Input: part model. Units: mm. Frame: model coordinates. Face numbers are marked on the shaded views. A direction names the side the tool comes from. Coordinates: 2 decimals unless noted, no trailing zeros. Order: outer loops, then holes, each group sorted by start corner. A loop starts at its lowest first (then second) coordinate and runs counter-clockwise, first axis right, second up. Notation, with made-up numbers: (40.5, -35.75) -> (47.5, -35.75) arc R15 cw to (47.5, -22.75) -> close; hole circle Ø1 at (51, 28). An arc over 180 degrees is marked (long way). Answer as CSV lines item,"result".
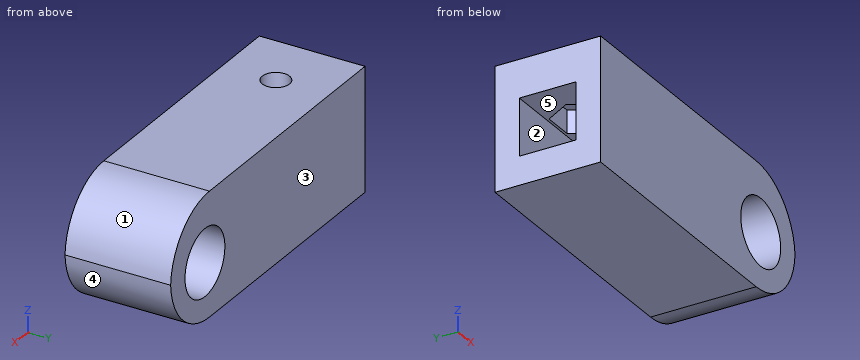
from build123d import *

# Parameters (mm, degrees)
ESBO_O2_R                = 4.1
RESSALTO_EXTRUS_O1_DEPTH = 13
ESBO_O3_W                = 7
ESBO_O3_H                = 7
CORTE_EXTRUS_O1_DEPTH    = 26
CORTE_EXTRUS_O2_DEPTH    = 2.8
ESBO_O10_R               = 1.683661958
CORTE_EXTRUS_O3_DEPTH    = 2.8
FILETE1_R                = 8


with BuildPart() as part:
    # Esboço2 → Ressalto-extrusão1 (new body)
    with BuildSketch(Plane(origin=(0, 0, 0), x_dir=(1, 0, 0), z_dir=(0, 1, 0))):
        Polygon((20, -5), (20, 7), (-20, 7), (-20, -5), (-20, -8.161034979), (20, -8.161034979), align=None)
        with Locations(Location((12.930574096, 0, 0), (0, 0, 90))):
            Circle(ESBO_O2_R, mode=Mode.SUBTRACT)
    extrude(amount=RESSALTO_EXTRUS_O1_DEPTH)

    # Esboço3 → Corte-extrusão1 (cut)
    with BuildSketch(Plane.ZY.offset(20)):
        with Locations((0, 6.5)):
            Rectangle(ESBO_O3_W, ESBO_O3_H)
    extrude(amount=-CORTE_EXTRUS_O1_DEPTH, mode=Mode.SUBTRACT)

    # Esboço7 → Corte-extrusão2 (cut)
    with BuildSketch(Plane(origin=(0, 0, 3.5), x_dir=(-1, 0, 0), z_dir=(0, 0, -1))):
        Polygon((8.882456985, 6.475905175), (10.729977846, 3.275905175), (14.425019569, 3.275905175), (16.272540431, 6.475905175), (14.425019569, 9.675905175), (10.729977846, 9.675905175), align=None)
    extrude(amount=-CORTE_EXTRUS_O2_DEPTH, mode=Mode.SUBTRACT)

    # Esboço10 → Corte-extrusão3 (cut)
    with BuildSketch(Plane(origin=(0, 0, 6.3), x_dir=(-1, 0, 0), z_dir=(0, 0, -1))):
        with Locations((12.577498708, 6.475905175)):
            Circle(ESBO_O10_R)
    extrude(amount=-CORTE_EXTRUS_O3_DEPTH, mode=Mode.SUBTRACT)

    # Filete1
    # the kernel refuses this fillet: 8 mm, written as the material it takes off along each edge
    with BuildSketch(Plane(origin=(20, -20, -7), x_dir=(0, 0, 1), z_dir=(0, 1, 0))) as filete1_piece_1:
        with BuildLine():
            CenterArc((FILETE1_R, -FILETE1_R), FILETE1_R, 90, 90)
            Line((0, -FILETE1_R), (0, 0))
            Line((0, 0), (FILETE1_R, 0))
        make_face()
    extrude(amount=53, mode=Mode.SUBTRACT)
    with BuildSketch(Plane(origin=(20, -20, 8.161034979), x_dir=(0, 0, -1), z_dir=(0, 1, 0))) as filete1_piece_2:
        with BuildLine():
            CenterArc((FILETE1_R, FILETE1_R), FILETE1_R, 180, 90)
            Line((0, FILETE1_R), (0, 0))
            Line((0, 0), (FILETE1_R, 0))
        make_face()
    extrude(amount=53, mode=Mode.SUBTRACT)


solid = part.part
1. Ray query, line 1 along Y through (x, z) = (-3.5, 1); line 2 along Z through (x, y) = (-4, 9.5); line 3 along X through (y, z) = (8.5, 3.75). Return the intervals inside material, ascending.
Findings:
line 1,"y = 0 to 3, 10 to 13"
line 2,"z = -7 to -3.5, 3.5 to 8.16"
line 3,"x = -20 to -15.1, -10.05 to 11.27, 14.59 to 19.15"
2. Cut plane A-A (z = -3). Return the cut outline in (x, y), plus the area to 3 significant figures.
Findings:
outline,"(-20, 0) -> (10.14, 0) -> (10.14, 13) -> (-20, 13) -> (-20, 10) -> (6, 10) -> (6, 3) -> (-20, 3) -> close; (15.73, 0) -> (18.93, 0) -> (18.93, 13) -> (15.73, 13) -> close"
area,"251 mm2"
3. Reachability of the marked faces 4 and 5 from +Z, -Z, +X, -X, +Y, -Y: full face, straight path, thin tool, end or side. Return the list, or none.
Findings:
face 4,"-Z, +X, +Y, -Y"
face 5,"-X"
4. Mould query, pull axis Y, two halves, no side actions, for the marked faces 1, 2 and 3. Classes: released by +Y, released by -Y, zero draft, split by the parting line, or undercut.
Findings:
face 1,"zero draft"
face 2,"undercut"
face 3,"released by +Y"
5. Cut plane B-B (x = -4). Return the cut outline in (y, z), plus the area to 3 significant figures.
Findings:
outline,"(0, -7) -> (13, -7) -> (13, 8.16) -> (0, 8.16) -> close; hole (3, -3.5) -> (10, -3.5) -> (10, 3.5) -> (3, 3.5) -> close"
area,"148 mm2"
6. Contact query for a flat-ended pin moving along its axis: pin 1 (6 mm diameter, centred on y = 6, z = -4, fed in from +X). Output: stop coordinate, or through.
Findings:
pin 1,"stops at x = 19.75"
7. Cut plane D-D (y = 8.75). Return the cut outline in (x, z), plus the area to 3 significant figures.
Findings:
outline,"(-20, -7) -> (12, -7) arc R8 ccw to (19.99, 0.58) arc R8 ccw to (12, 8.16) -> (-20, 8.16) -> (-20, 3.5) -> (-14.96, 3.5) -> (-14.96, 6.3) -> (-10.2, 6.3) -> (-10.2, 3.5) -> (6, 3.5) -> (6, -3.5) -> (-20, -3.5) -> close; hole circle Ø8.2 at (12.93, 0)"
area,"331 mm2"
8. Cut plane C-C (x = 11.5). Return the cut outline in (y, z).
Findings:
outline,"(0, -7) -> (13, -7) -> (13, -3.84) -> (0, -3.84) -> close; (0, 3.84) -> (13, 3.84) -> (13, 8.16) -> (0, 8.16) -> close"
